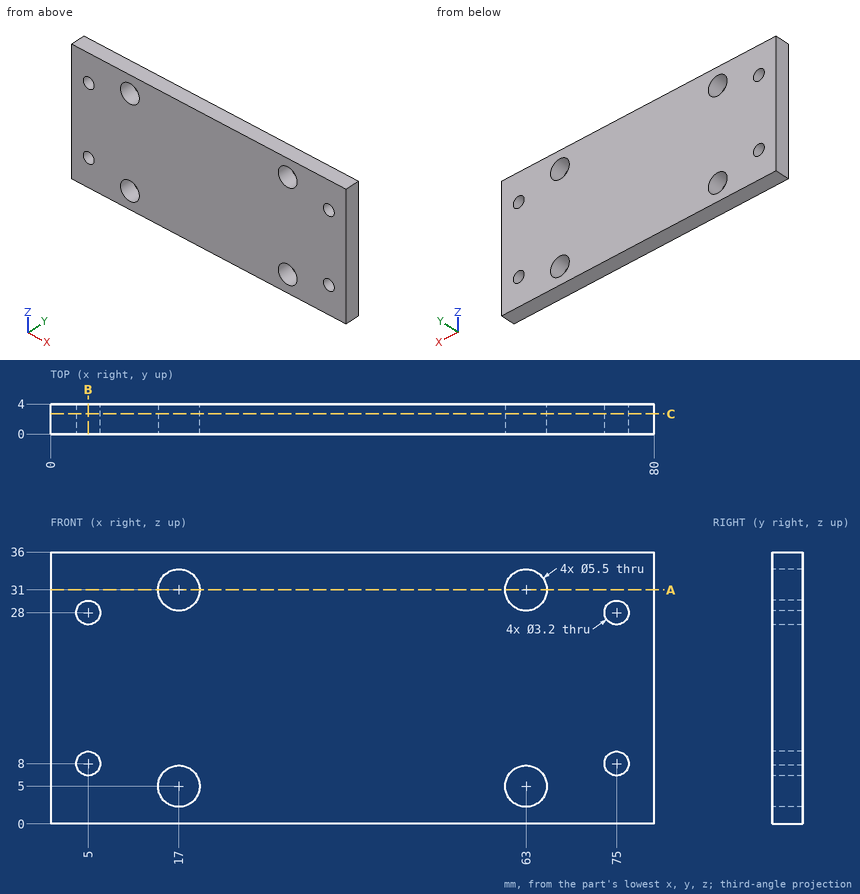
Part print with two shaded views. Sizes in mm from the minimum x, y, z corner. Coordinates: 2 decimals unless noted, no trailing zeros. Write each loop counter-clockwise with the first axis right and the second up, starting at its lowest first coordinate (ties: lowest second). Pieces come first, ordered by that corner, then holes. Notation, with made-up numbers: (68.25, -35) - (123.25, -35) arc R24 ccw to (123.25, 1) - close; hole circle Ø3 at (-36.75, 29). An arc over 180 degrees is marked (long way). One line per item, written item: value. Start each with the question number.
1. Slice it at C-C (y = 2.7). Count the separate pieces of the cut face and the enclosed holes in it, plus the area to 3 significant figures.
2. Slice it at B-B (x = 5). Write the cut outline in (y, z).
3. Probe line 1 (X direction, y = 2.2, z = 5); line 2 (Z direction, x = 75, y = 3.25); line 3 (X direction, y = 2.25, z = 8). List the from-to ranges inside material, lowest first. Write a range as from..to.
4. Flat gauge pin, fed straight in: pin 1 (5 mm diameter, centred on x = 5, z = 28, fed in from -Y). Where does the tip first touch, or does it go through?
5. Slice it at A-A (z = 31). Write the cut outline in (x, y), plus the area to 3 significant figures.
Answers below:
1. separate pieces: 1
1. enclosed holes: 8
1. area: 2,750 mm^2
2. outline: (0, 0) - (4, 0) - (4, 6.4) - (0, 6.4) - close; (0, 9.6) - (4, 9.6) - (4, 26.4) - (0, 26.4) - close; (0, 29.6) - (4, 29.6) - (4, 36) - (0, 36) - close
3. line 1: x = 0..14.25, 19.75..60.25, 65.75..80
3. line 2: z = 0..6.4, 9.6..26.4, 29.6..36
3. line 3: x = 0..3.4, 6.6..73.4, 76.6..80
4. pin 1: stops at y = 0
5. outline: (0, 0) - (14.25, 0) - (14.25, 4) - (0, 4) - close; (19.75, 0) - (60.25, 0) - (60.25, 4) - (19.75, 4) - close; (65.75, 0) - (80, 0) - (80, 4) - (65.75, 4) - close
5. area: 276 mm^2
